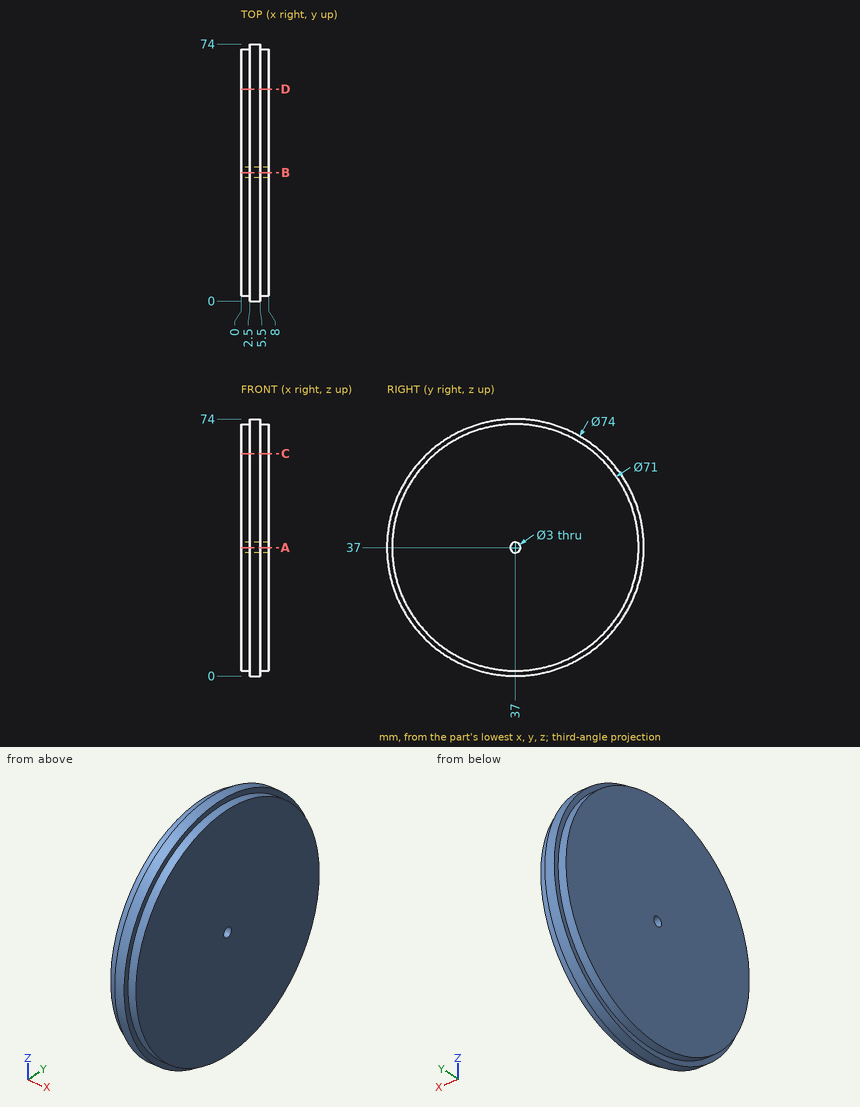
Verification items for this drawing (mm, ordinates from the low corner). Give positions to 0.01 mm unless a question says otherwise; leave off trailing zeros. Loops run counter-clockwise (first coordinate to the right, second up) from the corner with the lowest first, then second, coordinate; pieces in that order, holes last. Notation, with made-up numbers: M -33,-11 L -4,-11 A24 cw -4,24 Z; hole C 37.25,17.5 d2. An arc over 180 degrees is marked long. Answer as CSV lines item,"result".
Item 1: Cross-section at D-D on y = 61. Record the cut outline in (x, z), and give its area (3 significant figures).
Values:
outline,"M 0,10.84 L 2.5,10.84 L 2.5,8.84 L 5.5,8.84 L 5.5,10.84 L 8,10.84 L 8,63.16 L 5.5,63.16 L 5.5,65.16 L 2.5,65.16 L 2.5,63.16 L 0,63.16 Z"
area,"431 mm²"
Item 2: Cross-section at C-C on z = 64. Record the cut outline in (x, y).
Values:
outline,"M 0,13.95 L 2.5,13.95 L 2.5,11.7 L 5.5,11.7 L 5.5,13.95 L 8,13.95 L 8,60.05 L 5.5,60.05 L 5.5,62.3 L 2.5,62.3 L 2.5,60.05 L 0,60.05 Z"
Item 3: Material ranges on line 1 (Z direction, x = 3, y = 37); line 2 (X direction, y = 7, z = 56.5); line 3 (Y direction, x = 7.5, z = 9.5), recorded low to high.
Values:
line 1,"z = 0 to 35.5, 38.5 to 74"
line 2,"x = 2.5 to 5.5"
line 3,"y = 14.55 to 59.45"
Item 4: Depth check by flat-ended pin: P1, Ø1.5, axis at x = 6, z = 8, coming from the +Y side; P2, Ø2, axis at x = 4.5, z = 20.5, coming from the +Y side; P3, Ø1.5, axis at x = 1, y = 24.5, coming from the +Z side. Enter the tip coordinate at first touch or a pass-through.
Values:
P1,"stops at y = 60.67"
P2,"stops at y = 70.6"
P3,"stops at z = 70.5"
Item 5: Cross-section at A-A on z = 37. Record the cut outline in (x, y).
Values:
outline,"M 0,1.5 L 2.5,1.5 L 2.5,0 L 5.5,0 L 5.5,1.5 L 8,1.5 L 8,35.5 L 0,35.5 Z; M 0,38.5 L 8,38.5 L 8,72.5 L 5.5,72.5 L 5.5,74 L 2.5,74 L 2.5,72.5 L 0,72.5 Z"
